Autodesk Inventor part; units mm, degrees
ref_plane "YZ Plane" through (0, 0, 0) normal (1, 0, 0) x (0, 1, 0)
ref_plane "XZ Plane" through (0, 0, 0) normal (0, 1, 0) x (-1, 0, 0)
ref_plane "XY Plane" through (0, 0, 0) normal (0, 0, 1) x (1, 0, 0)
sketch "Sketch1" plane through (0, 0, 0) normal (0, 1, 0) x (-1, 0, 0)
  line L0 (0, 0) -> (30, 0)
  line L1 (30, 0) -> (30, -80)
  line L2 (30, -80) -> (0, -80)
  line L3 (0, -80) -> (0, 0)
  dimension "d0" = 30
  dimension "d1" = 80
extrude "Extrusion1" add sketch "Sketch1" along normal blind 7
fillet "Fillet1" radius 15 2 edges at (0, 3.5, -80) (-30, 3.5, -80)
sketch "Sketch2" plane through (0, 7, 0) normal (0, 1, 0) x (1, 0, 0)
  arc A0 (0, 65) -> (-30, 65) centre (-15, 65) ccw
  circle A1 centre (-15, 65) radius 5
  point P0 (0, 0)
  dimension "d5" = 10
extrude "Extrusion2" cut sketch "Sketch2" against normal blind 7
sketch "Sketch3" plane through (0, 0, 0) normal (0, -1, 0) x (1, 0, 0)
  line L0 (-30, 0) -> (0, 0)
  circle A0 centre (-15, -10) radius 2.7
  dimension "d9" = 5.4
extrude "Extrusion3" cut sketch "Sketch3" against normal blind 3
sketch "Sketch4" plane through (0, 7, 0) normal (0, 1, 0) x (1, 0, 0)
  line L0 (-30, 0) -> (0, 0)
  line L1 (-15, 0) -> (-15, 10)
  circle A0 centre (-15, 10) radius 1.5
  dimension "d12" = 10
  dimension "d13" = 3
extrude "Extrusion4" cut sketch "Sketch4" against normal blind 7
properties part number "Crank"
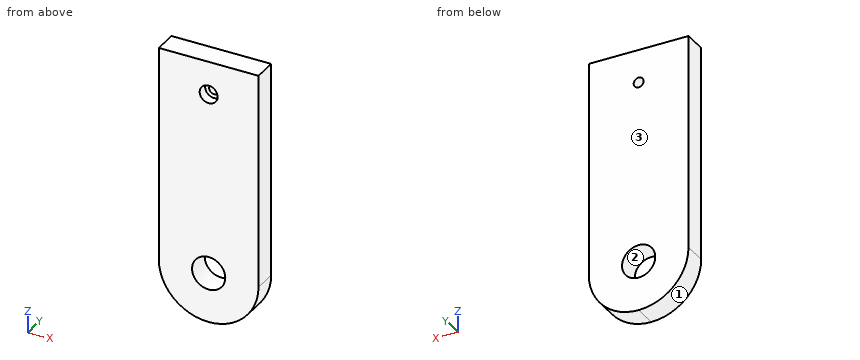
Input: part model. Units: mm. Frame: model coordinates. Face numbers are marked on the shaded views. Coordinates: 2 decimals unless noted, no trailing zeros. Order: outer loops, then holes, each group sorted by start corner. A loop starts at its lowest first (then second) coordinate and runs counter-clockwise, first axis right, second up.
1. Cut plane D-D, the plane x = -7.75. Return loops of the section in (y, z).
Checked values:
outline: (0, -78.13) - (7, -78.13) - (7, 0) - (0, 0) - close
2. Ray query, line 1 along Z through (x, y) = (-15, 5.5); line 2 along Z through (x, y) = (-15, 1.65); line 3 along X through (y, z) = (5.25, -65). Return the intervals inside material, ascending.
Checked values:
line 1: z = -80 to -70, -60 to -11.5, -8.5 to 0
line 2: z = -80 to -70, -60 to -12.7, -7.3 to 0
line 3: x = -30 to -20, -10 to 0
3. Cut plane A-A, the plane z = -10. Return loops of the section in (x, y), plus the area to 3 significant figures.
Checked values:
outline: (-30, 0) - (-17.7, 0) - (-17.7, 3) - (-16.5, 3) - (-16.5, 7) - (-30, 7) - close; (-13.5, 3) - (-12.3, 3) - (-12.3, 0) - (0, 0) - (0, 7) - (-13.5, 7) - close
area: 182 mm2
4. Draft query along X for the marked faces 1, 2 and 3. Return one class per face: +X half, -X half, draft (parallel to the pull), parting line (faces both ways), or undercut.
Checked values:
face 1: -X half
face 2: undercut
face 3: draft
5. Contact query for a flat-ended pin moving along its axis: P1, Ø5, axis at x = -18, z = -47.5, coming from the -Y side. Output: stop coordinate, or through.
Checked values:
P1: stops at y = 0
6. Cut plane C-C, the plane x = -18.75. Return loops of the section in (y, z), plus the area to 3 significant figures.
Checked values:
outline: (0, -79.52) - (7, -79.52) - (7, -68.31) - (0, -68.31) - close; (0, -61.69) - (7, -61.69) - (7, 0) - (0, 0) - close
area: 510 mm2
7. Cut plane B-B, the plane y = 4. Count the separate pieces of the cut face and the enclosed holes in it, plus the area to 3 significant figures.
Checked values:
separate pieces: 1
enclosed holes: 2
area: 2,220 mm2
